Autodesk Fusion 360 part; units mm, degrees
sketch "スケッチ1" plane through (0, 0, 0) normal (0, 0, 1) x (1, 0, 0)
  line L0 (0, 0) -> (20, 0)
  line L1 (20, 0) -> (20, 23)
  line L2 (20, 23) -> (0, 23)
  line L3 (0, 23) -> (0, 0)
  dimension "d1" = 20
  dimension "d2" = 23
extrude "押し出し1" add sketch "スケッチ1" along normal blind 2
sketch "スケッチ2" plane through (0, 0, 2) normal (0, 0, 1) x (-1, 0, 0)
  line L0 (0, -23) -> (0, 0)
  line L1 (0, 0) -> (-20, 0)
  line L2 (-20, 0) -> (-20, -23)
  line L3 (-20, -23) -> (0, -23)
  line L4 (0, -23) -> (-5, -23)
  line L5 (-5, -23) -> (-5, -18)
  line L6 (-5, -18) -> (0, -18)
  line L7 (0, -18) -> (0, -23)
  line L8 (-20, -23) -> (-15, -23)
  line L9 (-15, -23) -> (-15, -18)
  line L10 (-15, -18) -> (-20, -18)
  line L11 (-20, -18) -> (-20, -23)
  line L12 (0, 0) -> (-5, 0)
  line L13 (-5, 0) -> (-5, -5)
  line L14 (-5, -5) -> (0, -5)
  line L15 (0, -5) -> (0, 0)
  line L16 (-20, 0) -> (-15, 0)
  line L17 (-15, 0) -> (-15, -5)
  line L18 (-15, -5) -> (-20, -5)
  line L19 (-20, -5) -> (-20, 0)
  line L20 (-2, -21) -> (-18, -21)
  line L21 (-18, -21) -> (-18, -2)
  line L22 (-18, -2) -> (-2, -2)
  line L23 (-2, -2) -> (-2, -21)
  dimension "d5" = 5
  dimension "d6" = 5
  dimension "d7" = 5
  dimension "d8" = 5
  dimension "d9" = 5
  dimension "d10" = 5
  dimension "d11" = 5
  dimension "d12" = 5
extrude "押し出し2" add sketch "スケッチ2" along normal blind 2 contours L0 L3 L4 L5 L6 L7 L20 L23 | L0 L1 L12 L13 L14 L15 L22 L23 | L5 L6 L20 L23 | L5 L6 L9 L10 L13 L14 L17 L18 L20 L21 L22 L23 | L2 L3 L8 L9 L10 L11 L20 L21 | L13 L14 L22 L23 | L9 L10 L20 L21 | L1 L2 L16 L17 L18 L19 L21 L22 | L17 L18 L21 L22
sketch "スケッチ3" plane through (0, 0, 4) normal (0, 0, 1) x (-1, 0, 0)
  line L0 (-18, -18) -> (-20, -18)
  line L1 (-20, -18) -> (-20, -23)
  line L2 (-20, -23) -> (-15, -23)
  line L3 (-15, -23) -> (-15, -21)
  line L4 (-15, -21) -> (-5, -21)
  line L5 (-5, -21) -> (-5, -23)
  line L6 (-5, -23) -> (0, -23)
  line L7 (0, -23) -> (0, -18)
  line L8 (0, -18) -> (-2, -18)
  line L9 (-2, -18) -> (-2, -5)
  line L10 (-2, -5) -> (0, -5)
  line L11 (0, -5) -> (0, 0)
  line L12 (0, 0) -> (-5, 0)
  line L13 (-5, 0) -> (-5, -2)
  line L14 (-5, -2) -> (-15, -2)
  line L15 (-15, -2) -> (-15, 0)
  line L16 (-15, 0) -> (-20, 0)
  line L17 (-20, 0) -> (-20, -5)
  line L18 (-20, -5) -> (-18, -5)
  line L19 (-18, -5) -> (-18, -18)
  line L20 (-5, -18) -> (-15, -18)
  line L21 (-15, -18) -> (-15, -5)
  line L22 (-15, -5) -> (-5, -5)
  line L23 (-5, -5) -> (-5, -18)
extrude "押し出し3" add sketch "スケッチ3" along normal blind 3 contours L20 L21 L22 L23
sketch "スケッチ4" plane through (0, 0, 7) normal (0, 0, 1) x (-1, 0, 0)
  line L0 (-5, -5) -> (-15, -5)
  line L1 (-15, -5) -> (-15, -18)
  line L2 (-15, -18) -> (-5, -18)
  line L3 (-5, -18) -> (-5, -5)
  line L4 (-9.55, -13.5) -> (-11.05, -13.5)
  line L5 (-11.05, -13.5) -> (-11.05, -9.5)
  line L6 (-11.05, -9.5) -> (-9.55, -9.5)
  line L7 (-9.55, -9.5) -> (-9.55, -13.5)
  line L8 (-8.3, -12.25) -> (-12.3, -12.25)
  line L9 (-12.3, -12.25) -> (-12.3, -10.75)
  line L10 (-12.3, -10.75) -> (-8.3, -10.75)
  line L11 (-8.3, -10.75) -> (-8.3, -12.25)
  circle A0 centre (-10.3, -11.5) radius 2.75
  dimension "d17" = 13
  dimension "d18" = 1.5
  dimension "d19" = 4
  dimension "d20" = 4
  dimension "d21" = 1.5
  dimension "d22" = 5.5
extrude "押し出し4" add sketch "スケッチ4" along normal blind 3.5 contours A0
sketch "スケッチ5" plane through (0, 0, 0) normal (0, 0, -1) x (1, 0, 0)
  line L0 (0, 0) -> (0, -23)
  line L1 (0, -23) -> (20, -23)
  line L2 (20, -23) -> (20, 0)
  line L3 (20, 0) -> (0, 0)
  line L4 (4, -12) -> (4, -14)
  line L5 (4, -12) -> (4, -11)
  line L6 (13, -11) -> (13, -12)
  line L7 (5, -12) -> (4, -12)
  line L8 (5, -14) -> (5, -12)
  line L9 (4, -14) -> (5, -14)
  line L10 (4, -11) -> (13, -11)
  line L11 (13, -12) -> (4, -12)
  line L12 (13, -11) -> (13, -9)
  line L13 (13, -9) -> (16, -11.5)
  line L14 (16, -11.5) -> (13, -14)
  line L15 (13, -14) -> (13, -12)
extrude "押し出し5" cut sketch "スケッチ5" against normal blind 1 contours L4 L7 L8 L9 L11 | L5 L6 L7 L10 L11 | L6 L12 L13 L14 L15
Source: CAD feature listing. Evaluate the final solid. Frame: model axes, mm. A direction names the side the tool comes from. Round coordinates to 2 decimals unless told otherwise and drop trailing zeros. Write each loop counter-clockwise with the first axis right and the second up, starting at its lowest first coordinate (ties: lowest second). Pieces come first, ordered by that corner, then holes. Notation, with made-up numbers: M -7,-20 L 26,-20 A19 ccw 26,-8 Z; hole C 47.25,-9.5 d1. An arc over 180 degrees is marked long. Use CSV: the item, a comma, the result in double quotes. Start each with the question number.
Q1. Pull-direction query (X, two-part tool) for faces 4 (the face through (9.55, 13, 9)), 5 (the face through (2, 11, 3)), 6 (the face through (10.1, 23, 1.5)); classes: +X half, -X half, draft (parallel to the pull), parting line (faces both ways), or undercut.
Q2. Cut plane A-A on z = 9.5. Output: boundary loops of the cut face in (x, y), plus the area to 3 significant figures.
Q3. First-contact query: P1, Ø1.1, axis at x = 8, z = 0.5, coming from the -Y side; P2, Ø6, axis at x = 14.5, y = 20, coming from the +Z side; P3, Ø0.6, axis at y = 10, z = 8.5, coming from the -X side; P4, Ø1, axis at y = 15.5, z = 4, coming from the -X side. Flat tips, straight axial feed; report the tip coordinate or a pass-through.
Q4. Line query: line 1 (Z direction, x = 7.5, y = 16.75); line 2 (Z direction, x = 15.5, y = 18); line 3 (X direction, y = 13.5, z = 5). Output: solid intervals per line, ascending. Write a range as from..to.
Q5. Access query for faces 1 (the face through (13, 13, 0.5)), 2 (the face through (18, 12, 3)), 3 (the face through (9, 10.75, 9)). Directions: +Z, -Z, +X, -X, +Y, -Y. A direction counts if a zero-diameter tool reaches every point of the face in a straight line with its end or side. Return the directions, or none.
Q6. Cut plane D-D on y = 21.5. Output: boundary loops of the cut face in (x, z).
Q7. Cut plane B-B on x = 6.5. Output: boundary loops of the cut face in (y, z).
Q8. Cut plane C-C on y = 15.75. Output: boundary loops of the cut face in (x, z).
Results found:
1,face 4,"undercut"
1,face 5,"-X half"
1,face 6,"draft"
2,outline,"C 10.3,11.5 d5.5; hole M 8.3,10.75 L 9.55,10.75 L 9.55,9.5 L 11.05,9.5 L 11.05,10.75 L 12.3,10.75 L 12.3,12.25 L 11.05,12.25 L 11.05,13.5 L 9.55,13.5 L 9.55,12.25 L 8.3,12.25 Z"
2,area,"14.0 mm^2"
3,P1,"y = 0"
3,P2,"z = 7"
3,P3,"x = 7.83"
3,P4,"x = 2"
4,line 1,"0..7"
4,line 2,"0..4"
4,line 3,"5..15"
5,face 1,"-Z"
5,face 2,"+Z, +X"
5,face 3,"+Z"
6,outline,"M 0,0 L 20,0 L 20,4 L 15,4 L 15,2 L 5,2 L 5,4 L 0,4 Z"
7,outline,"M 0,0 L 11,0 L 11,1 L 12,1 L 12,0 L 23,0 L 23,2 L 21,2 L 21,4 L 18,4 L 18,7 L 5,7 L 5,4 L 2,4 L 2,2 L 0,2 Z"
8,outline,"M 0,0 L 20,0 L 20,2 L 18,2 L 18,4 L 15,4 L 15,7 L 5,7 L 5,4 L 2,4 L 2,2 L 0,2 Z"
